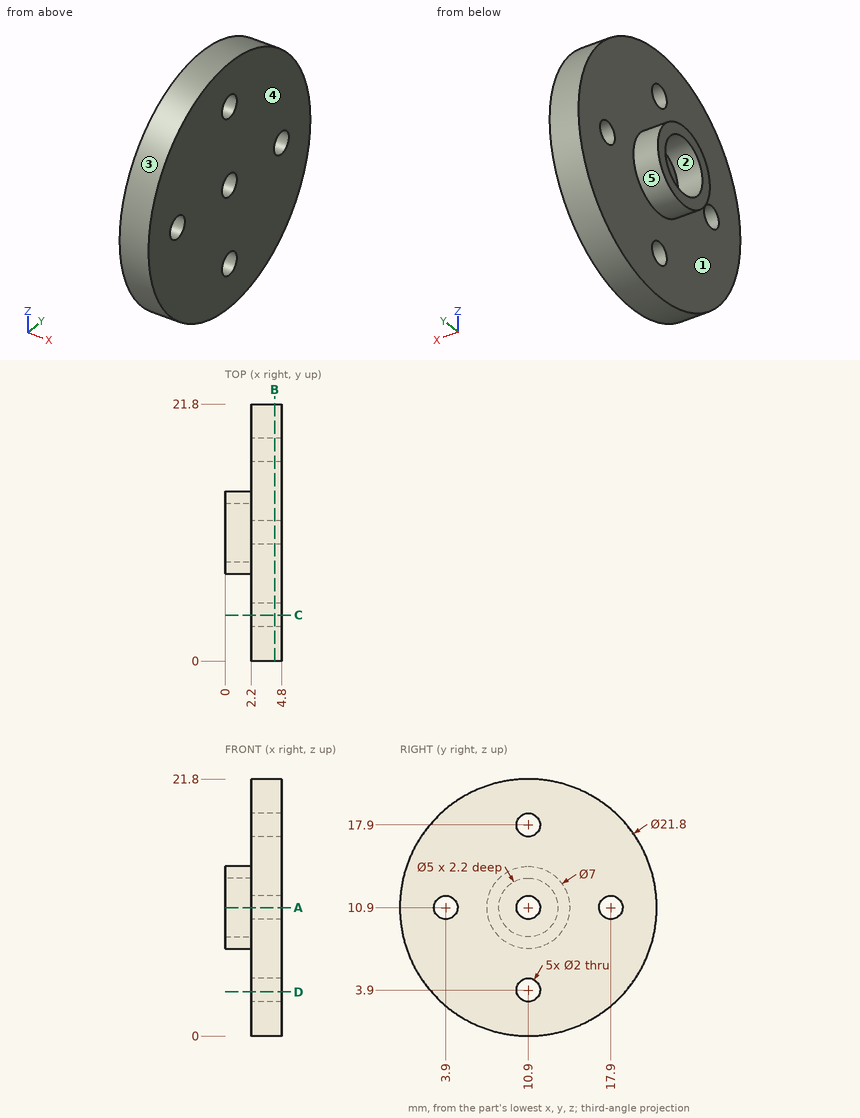
Design review of the part shown in the three views and the two pictorial views. Dimensions are in mm from the part's minimum x, y and z. A direction names the side the tool comes from. Round coordinates to 2 decimals unless told otherwise and drop trailing zeros. Write each loop counter-clockwise with the first axis right and the second up, starting at its lowest first coordinate (ties: lowest second). Pieces come first, ordered by that corner, then holes. Notation, with made-up numbers: (38, 72.25) -> (63, 72.25) arc R26 ccw to (63, 89.25) -> close; hole circle Ø10 at (78.5, -4). An arc over 180 degrees is marked (long way). Use one line per item in the form item = value.
1) Take a section at C-C, the plane y = 3.9. Write out the cut boundary in (x, z), and give its area (3 significant figures).
Found:
outline = (2.2, 2.54) -> (4.8, 2.54) -> (4.8, 9.9) -> (2.2, 9.9) -> close; (2.2, 11.9) -> (4.8, 11.9) -> (4.8, 19.26) -> (2.2, 19.26) -> close
area = 38.2 mm2
2) Take a section at D-D, the plane z = 3.75. Write out the cut boundary in (x, y), and give its area (3 significant figures).
Found:
outline = (2.2, 2.67) -> (4.8, 2.67) -> (4.8, 9.91) -> (2.2, 9.91) -> close; (2.2, 11.89) -> (4.8, 11.89) -> (4.8, 19.13) -> (2.2, 19.13) -> close
area = 37.6 mm2
3) To check wall thickness, follow L1, parallel to Z at x = 4.25, y = 10.9; L2, parallel to X at y = 9.25, z = 10.5; L3, parallel to Y at x = 1.65, z = 10.9. State the ranges of each line that lie inside material, in increasing order. Write a range as from..to.
Found:
L1 = 0..2.9, 4.9..9.9, 11.9..16.9, 18.9..21.8
L2 = 2.2..4.8
L3 = 7.4..8.4, 13.4..14.4
4) Tool access review of the marked faces 4 and 5: name each direction out of +Z, -Z, +X, -X, +Y, -Y from which nothing blocks a thin tool from reaching the whole face with its end or side.
Found:
face_4 = +Z, -Z, +X, +Y, -Y
face_5 = -X
5) Clearance check with flat-ended pins moving along their axes: pin 1 (5.5 mm diameter, centred on y = 11.5, z = 12, fed in from -X); pin 2 (1.8 mm diameter, centred on y = 10.9, z = 3.9, fed in from +X); pin 3 (5 mm diameter, centred on y = 4.5, z = 17, fed in from -X); pin 4 (2 mm diameter, centred on x = 2.5, y = 15.5, fed in from +Z). State where each tip first meets the part, or that it passes through.
Found:
pin_1 = 0
pin_2 = through
pin_3 = 2.2
pin_4 = 21.19
6) Take a section at A-A, the plane z = 10.9. Write out the cut boundary in (x, y).
Found:
outline = (0, 7.4) -> (2.2, 7.4) -> (2.2, 4.9) -> (4.8, 4.9) -> (4.8, 9.9) -> (2.2, 9.9) -> (2.2, 8.4) -> (0, 8.4) -> close; (0, 13.4) -> (2.2, 13.4) -> (2.2, 11.9) -> (4.8, 11.9) -> (4.8, 16.9) -> (2.2, 16.9) -> (2.2, 14.4) -> (0, 14.4) -> close; (2.2, 0) -> (4.8, 0) -> (4.8, 2.9) -> (2.2, 2.9) -> close; (2.2, 18.9) -> (4.8, 18.9) -> (4.8, 21.8) -> (2.2, 21.8) -> close
7) Take a section at B-B, the plane x = 4.2. Write out the cut boundary in (y, z), and give its area (3 significant figures).
Found:
outline = circle Ø21.8 at (10.9, 10.9); hole circle Ø2 at (3.9, 10.9); hole circle Ø2 at (10.9, 3.9); hole circle Ø2 at (10.9, 10.9); hole circle Ø2 at (10.9, 17.9); hole circle Ø2 at (17.9, 10.9)
area = 358 mm2
8) Mouldability with a two-part tool opening along Z and no side actions: class the marked faces 1, 2 and 3 as +Z half, -Z half, draft (parallel to the pull), parting line (faces both ways), or undercut.
Found:
face_1 = draft
face_2 = undercut
face_3 = parting line
